Read the model definition and answer for the solid it produces. Units are mm, in the model's axes. A direction names the side the tool comes from. Give positions to 0.01 mm unless a question says otherwise; leave off trailing zeros. Write each loop counter-clockwise with the first axis right and the second up, starting at its lowest first coordinate (ties: lowest second). Pieces come first, ordered by that corner, then holes. Notation, with made-up numbers: (26, -5) - (31, -5) arc R7 cw to (31, 1) - close; hole circle Ø4 at (51, 6). An arc over 180 degrees is marked (long way). Use CSV: the item, a comma, the result in double quotes. Start each with the question number.
from build123d import *

# Parameters (mm, degrees)
SKETCH1_R           = 10
SKETCH1_W           = 30
SKETCH1_H           = 3
BOSS_EXTRUDE1_DEPTH = 3
BOSS_EXTRUDE3_DEPTH = 5
SKETCH2_W           = 22.5
SKETCH2_H           = 34
BOSS_EXTRUDE2_DEPTH = 2
SKETCH4_R           = 1.6
CUT_EXTRUDE1_DEPTH  = 11
FILLET1_R           = 3


with BuildPart() as part:
    # Sketch1 → Boss-Extrude1 (new body)
    with BuildSketch(Plane.XY):
        with BuildLine():
            Line((-150, 98.203720637), (-150, 69.203720637))
            ThreePointArc((-150, 69.203720637), (-149.267766953, 67.435953684), (-147.5, 66.703720637))
            Line((-147.5, 66.703720637), (-78.5, 66.703720637))
            ThreePointArc((-78.5, 66.703720637), (-76.732233047, 67.435953684), (-76, 69.203720637))
            Line((-76, 69.203720637), (-76, 98.203720637))
            ThreePointArc((-76, 98.203720637), (-76.732233047, 99.97148759), (-78.5, 100.703720637))
            Line((-78.5, 100.703720637), (-147.5, 100.703720637))
            ThreePointArc((-147.5, 100.703720637), (-149.267766953, 99.97148759), (-150, 98.203720637))
        make_face()
        with Locations((-130.886316496, 83.527802162)):
            Circle(SKETCH1_R, mode=Mode.SUBTRACT)
        with Locations((-97.886316496, 83.703720637)):
            Rectangle(SKETCH1_W, SKETCH1_H, mode=Mode.SUBTRACT)
        with Locations((-97.886316496, 88.703720637)):
            Rectangle(SKETCH1_W, SKETCH1_H, mode=Mode.SUBTRACT)
        with Locations((-97.886316496, 78.703720637)):
            Rectangle(SKETCH1_W, SKETCH1_H, mode=Mode.SUBTRACT)
    extrude(amount=-BOSS_EXTRUDE1_DEPTH)

    # Sketch3 → Boss-Extrude3 (add)
    with BuildSketch(Plane(origin=(0, 0, -3), x_dir=(-1, 0, 0), z_dir=(0, 0, -1))):
        with BuildLine():
            Line((150, 98.203720637), (150, 69.203720637))
            ThreePointArc((150, 69.203720637), (149.267766953, 67.435953684), (147.5, 66.703720637))
            Line((147.5, 66.703720637), (147.5, 100.703720637))
            ThreePointArc((147.5, 100.703720637), (149.267766953, 99.97148759), (150, 98.203720637))
        make_face()
        with BuildLine():
            Line((78.5, 100.703720637), (78.5, 66.703720637))
            ThreePointArc((78.5, 66.703720637), (76.732233047, 67.435953684), (76, 69.203720637))
            Line((76, 69.203720637), (76, 98.203720637))
            ThreePointArc((76, 98.203720637), (76.732233047, 99.97148759), (78.5, 100.703720637))
        make_face()
    extrude(amount=BOSS_EXTRUDE3_DEPTH)

    # Sketch2 → Boss-Extrude2 (add)
    with BuildSketch(Plane(origin=(0, 0, -8), x_dir=(-1, 0, 0), z_dir=(0, 0, -1))):
        with Locations((158.75, 83.703720637)):
            Rectangle(SKETCH2_W, SKETCH2_H)
        with Locations((67.25, 83.703720637)):
            Rectangle(SKETCH2_W, SKETCH2_H)
    extrude(amount=BOSS_EXTRUDE2_DEPTH)

    # Sketch4 → Cut-Extrude1 (cut, through all)
    with BuildSketch(Plane(origin=(0, 0, -10), x_dir=(-1, 0, 0), z_dir=(0, 0, -1))):
        with Locations((61, 93.703720637)):
            Circle(SKETCH4_R)
        with Locations((61, 73.703720637)):
            Circle(SKETCH4_R)
        with Locations((165, 73.703720637)):
            Circle(SKETCH4_R)
        with Locations((165, 93.703720637)):
            Circle(SKETCH4_R)
    extrude(amount=-CUT_EXTRUDE1_DEPTH, mode=Mode.SUBTRACT)

    # Fillet1
    fillet1_edges = [part.edges().sort_by_distance(p)[0] for p in [
        (-56, 100.703720637, -9),
        (-56, 66.703720637, -9),
        (-170, 66.703720637, -9),
        (-170, 100.703720637, -9),
    ]]
    fillet(fillet1_edges, radius=FILLET1_R)


solid = part.part
(1) For a pull along Y with two mould halves and no side action, classify faces 1 (the face through (-56.9, 67.56, -9.01)), 2 (the face through (-159, 84, -8)), 3 (the face through (-157, 100.704, -9)), 4 (the face through (-98, 77.204, -1)) as pulls with the +Y half, pulls with the -Y half, needs draft (parallel to the pull), parting line crosses it, or undercut.
(2) The part is cut by section C-C on y = 78.5. Write down the section's boundary in (x, z), plus the area to 3 significant figures.
(3) Which of the six approach directions +Z, -Z, +X, -X, +Y, -Y give full straight-line access (tool end or side, diameter ignored) to faces 5 (the face through (-82.886, 84, -1)), 6 (the face through (-149.25, 99.99, -3.94)), 7 (the face through (-170, 84, -9))?
(4) The part is cut by section D-D on x = -165. Write down the section's boundary in (y, z), plus the area to 3 significant figures.
(5) Consider probe 1 along Y at (x, z) = (-61, -8.9); probe 2 along Y at (x, z) = (-102.5, -2.75); probe 3 along X at (y, z) = (77, -5.75). Determine where each line is inside the solid, lowest interval first.
(6) The part is cut by section B-B on z = -4. Write down the section's boundary in (x, y).
(7) The part is cut by section A-A on x = -100.5. Write down the section's boundary in (y, z).
(8) Given P1, Ø3.5, axis at y = 89, z = -2, coming from the -X side; P2, Ø2, axis at y = 83, z = -6.5, coming from the +X side; P3, Ø11, axis at x = -163, y = 92, coming from the +Z side, each flat-ended and moving along its own axis, determine where each tip first touches the part or whether it passes through.
Reported:
1,face 1,"pulls with the -Y half"
1,face 2,"needs draft"
1,face 3,"pulls with the +Y half"
1,face 4,"undercut"
2,outline,"(-170, -10) - (-147.5, -10) - (-147.5, -3) - (-139.53, -3) - (-139.53, 0) - (-150, 0) - (-150, -8) - (-170, -8) - close; (-122.24, -3) - (-112.89, -3) - (-112.89, 0) - (-122.24, 0) - close; (-82.89, -3) - (-78.5, -3) - (-78.5, -10) - (-56, -10) - (-56, -8) - (-76, -8) - (-76, 0) - (-82.89, 0) - close"
2,area,"195 mm²"
3,face 5,"+Z, -Z"
3,face 6,"+Z, -X, +Y"
3,face 7,"+Z, -Z, -X, +Y, -Y"
4,outline,"(66.7, -10) - (72.1, -10) - (72.1, -8) - (66.7, -8) - close; (75.3, -10) - (92.1, -10) - (92.1, -8) - (75.3, -8) - close; (95.3, -10) - (100.7, -10) - (100.7, -8) - (95.3, -8) - close"
4,area,"55.2 mm²"
5,probe 1,"66.7 to 72.1, 75.3 to 92.1, 95.3 to 100.7"
5,probe 2,"66.7 to 77.2, 80.2 to 82.2, 85.2 to 87.2, 90.2 to 100.7"
5,probe 3,"-150 to -147.5, -78.5 to -76"
6,outline,"(-150, 69.2) arc R2.5 ccw to (-147.5, 66.7) - (-147.5, 100.7) arc R2.5 ccw to (-150, 98.2) - close; (-78.5, 66.7) arc R2.5 ccw to (-76, 69.2) - (-76, 98.2) arc R2.5 ccw to (-78.5, 100.7) - close"
7,outline,"(66.7, -3) - (77.2, -3) - (77.2, 0) - (66.7, 0) - close; (80.2, -3) - (82.2, -3) - (82.2, 0) - (80.2, 0) - close; (85.2, -3) - (87.2, -3) - (87.2, 0) - (85.2, 0) - close; (90.2, -3) - (100.7, -3) - (100.7, 0) - (90.2, 0) - close"
8,P1,"x = -150"
8,P2,"x = -76"
8,P3,"z = -8"
